```python
from build123d import *

# Parameters (mm, degrees)
SKETCH1_W               = 40
SKETCH1_H               = 35
BOSS_EXTRUDE1_DEPTH     = 8
CUT_EXTRUDE1_DEPTH      = 1
CUT_EXTRUDE1_DEPTH_BACK = 41
FILLET1_R               = 2
SKETCH6_R               = 2
BOSS_EXTRUDE2_DEPTH     = 5
CUT_EXTRUDE2_DEPTH      = 7.467619242
SKETCH6_7_R             = 4.25
CUT_EXTRUDE3_DEPTH      = 3
SKETCH7_W               = 10
SKETCH7_H               = 3
CUT_EXTRUDE4_DEPTH      = 3
FILLET2_R               = 1
SKETCH8_W               = 20
SKETCH8_H               = 2
CUT_EXTRUDE5_DEPTH      = 36
SKETCH10_R              = 4.25
SKETCH10_R_2            = 2
SKETCH10_R_3            = 9
CUT_EXTRUDE6_DEPTH      = 3
FILLET3_R               = 0.5
SKETCH5_W               = 35
SKETCH5_H               = 2
BOSS_EXTRUDE3_DEPTH     = 10
SKETCH12_R              = 2
CUT_EXTRUDE7_DEPTH      = 7.467619242


with BuildPart() as part:
    # Sketch1 → Boss-Extrude1 (new body)
    with BuildSketch(Plane(origin=(0, 0, 0), x_dir=(1, 0, 0), z_dir=(0, 1, 0))):
        Rectangle(SKETCH1_W, SKETCH1_H)
    extrude(amount=-BOSS_EXTRUDE1_DEPTH)

    # Sketch2 → Cut-Extrude1 (cut, two sides)
    with BuildSketch(Plane(origin=(20, 0, 0), x_dir=(0, 0, -1), z_dir=(1, 0, 0))) as cut_extrude1_sk:
        Polygon((-12.5, -5), (-17.5, -8), (0, -8), (0, -5), align=None)
        Polygon((0, -5), (0, -8), (17.5, -8), (12.5, -5), align=None)
    extrude(amount=CUT_EXTRUDE1_DEPTH, mode=Mode.SUBTRACT)
    extrude(cut_extrude1_sk.sketch, amount=-CUT_EXTRUDE1_DEPTH_BACK, mode=Mode.SUBTRACT)

    # Fillet1
    fillet1_edges = [part.edges().sort_by_distance(p)[0] for p in [
        (0, -8, -17.5),
        (0, -5, 12.5),
        (0, -5, -12.5),
        (0, -8, 17.5),
    ]]
    fillet(fillet1_edges, radius=FILLET1_R)

    # Sketch6 → Boss-Extrude2 (add)
    with BuildSketch(Plane(origin=(0, 0, 0), x_dir=(1, 0, 0), z_dir=(0, 1, 0))):
        with BuildLine():
            Line((20, 17.5), (20, -17.5))
            Line((20, -17.5), (40, -17.5))
            ThreePointArc((40, -17.5), (57.5, 0), (40, 17.5))
            Line((40, 17.5), (20, 17.5))
        make_face()
        with Locations((40, -12)):
            Circle(SKETCH6_R, mode=Mode.SUBTRACT)
        with BuildLine():
            ThreePointArc((37.420408929, -8.622395833), (40, -7.75), (42.579591071, -8.622395833))
            ThreePointArc((42.579591071, -8.622395833), (40, -9), (37.420408929, -8.622395833))
        make_face(mode=Mode.SUBTRACT)
        with BuildLine():
            ThreePointArc((31.377604167, -2.579591071), (31, 0), (31.377604167, 2.579591071))
            ThreePointArc((31.377604167, 2.579591071), (32.025997871, 1.361558352), (32.25, 0))
            ThreePointArc((32.25, 0), (32.025997871, -1.361558352), (31.377604167, -2.579591071))
        make_face(mode=Mode.SUBTRACT)
        with BuildLine():
            ThreePointArc((37.420408929, 8.622395833), (40, 9), (42.579591071, 8.622395833))
            ThreePointArc((42.579591071, 8.622395833), (40, 7.75), (37.420408929, 8.622395833))
        make_face(mode=Mode.SUBTRACT)
        with Locations((40, 12)):
            Circle(SKETCH6_R, mode=Mode.SUBTRACT)
        with BuildLine():
            ThreePointArc((48.622395833, -2.579591071), (47.75, 0), (48.622395833, 2.579591071))
            ThreePointArc((48.622395833, 2.579591071), (49, 0), (48.622395833, -2.579591071))
        make_face(mode=Mode.SUBTRACT)
    extrude(amount=-BOSS_EXTRUDE2_DEPTH)

    # Sketch6<6> → Cut-Extrude2 (cut, through all)
    with BuildSketch(Plane(origin=(0, 0, 0), x_dir=(1, 0, 0), z_dir=(0, 1, 0))):
        with BuildLine():
            ThreePointArc((37.420408929, 8.622395833), (33.636038969, 6.363961031), (31.377604167, 2.579591071))
            ThreePointArc((31.377604167, 2.579591071), (32.025997871, 1.361558352), (32.25, 0))
            ThreePointArc((32.25, 0), (32.025997871, -1.361558352), (31.377604167, -2.579591071))
            ThreePointArc((31.377604167, -2.579591071), (33.636038969, -6.363961031), (37.420408929, -8.622395833))
            ThreePointArc((37.420408929, -8.622395833), (40, -7.75), (42.579591071, -8.622395833))
            ThreePointArc((42.579591071, -8.622395833), (46.363961031, -6.363961031), (48.622395833, -2.579591071))
            ThreePointArc((48.622395833, -2.579591071), (47.75, 0), (48.622395833, 2.579591071))
            ThreePointArc((48.622395833, 2.579591071), (46.363961031, 6.363961031), (42.579591071, 8.622395833))
            ThreePointArc((42.579591071, 8.622395833), (40, 7.75), (37.420408929, 8.622395833))
        make_face()
    extrude(amount=-CUT_EXTRUDE2_DEPTH, mode=Mode.SUBTRACT)

    # Sketch6<7> → Cut-Extrude3 (cut)
    with BuildSketch(Plane(origin=(0, 0, 0), x_dir=(1, 0, 0), z_dir=(0, 1, 0))):
        with Locations((52, 0)):
            Circle(SKETCH6_7_R)
        with Locations((28, 0)):
            Circle(SKETCH6_7_R)
    extrude(amount=-CUT_EXTRUDE3_DEPTH, mode=Mode.SUBTRACT)

    # Sketch7 → Cut-Extrude4 (cut)
    with BuildSketch(Plane(origin=(0, 0, 0), x_dir=(1, 0, 0), z_dir=(0, 1, 0))):
        with Locations((29, -16)):
            Rectangle(SKETCH7_W, SKETCH7_H)
    extrude(amount=-CUT_EXTRUDE4_DEPTH, mode=Mode.SUBTRACT)

    # Fillet2
    fillet2_edges = [part.edges().sort_by_distance(p)[0] for p in [
        (34, -1.5, 17.5),
    ]]
    fillet(fillet2_edges, radius=FILLET2_R)

    # Sketch8 → Cut-Extrude5 (cut, through all)
    with BuildSketch(Plane.XY.offset(17.5)):
        with Locations((12, -1)):
            Rectangle(SKETCH8_W, SKETCH8_H)
    extrude(amount=-CUT_EXTRUDE5_DEPTH, mode=Mode.SUBTRACT)

    # Sketch10 → Cut-Extrude6 (cut)
    with BuildSketch(Plane.XZ.offset(5)):
        with Locations((40, -12)):
            Circle(SKETCH10_R)
        with Locations((40, -12)):
            Circle(SKETCH10_R_2, mode=Mode.SUBTRACT)
        with Locations((40, 0)):
            Circle(SKETCH10_R_3)
        with Locations((40, 12)):
            Circle(SKETCH10_R)
        with Locations((40, 12)):
            Circle(SKETCH10_R_2, mode=Mode.SUBTRACT)
        with Locations((40, 0)):
            Circle(SKETCH10_R_3)
    extrude(amount=-CUT_EXTRUDE6_DEPTH, mode=Mode.SUBTRACT)

    # Fillet3
    fillet3_edges = [part.edges().sort_by_distance(p)[0] for p in [
        (49, -5, 0),
        (40, -5, -16.25),
        (40, -5, 16.25),
        (31, -5, 0),
    ]]
    fillet(fillet3_edges, radius=FILLET3_R)

    # Sketch5 → Boss-Extrude3 (add)
    with BuildSketch(Plane.ZY.offset(20)):
        with Locations((0, -1)):
            Rectangle(SKETCH5_W, SKETCH5_H)
    extrude(amount=BOSS_EXTRUDE3_DEPTH)

    # Sketch12 → Cut-Extrude7 (cut, through all)
    with BuildSketch(Plane(origin=(0, 0, 0), x_dir=(1, 0, 0), z_dir=(0, 1, 0))):
        with Locations((-25, 12)):
            Circle(SKETCH12_R)
        with Locations((-25, -12)):
            Circle(SKETCH12_R)
    extrude(amount=-CUT_EXTRUDE7_DEPTH, mode=Mode.SUBTRACT)


solid = part.part
```
Input: part model. Units: mm. Frame: model coordinates. A direction names the side the tool comes from. Coordinates: 2 decimals unless noted, no trailing zeros. Order: outer loops, then holes, each group sorted by start corner. A loop starts at its lowest first (then second) coordinate and runs counter-clockwise, first axis right, second up. Notation, with made-up numbers: (81.5, 70) - (90.5, 70) arc R9 ccw to (90.5, 78) - close; hole circle Ø1 at (-26.5, -0.5). An arc over 180 degrees is marked (long way). Put each result on its own line as item: value.
1. Line query: line 1 along Z through (x, y) = (40, -4); line 2 along Z through (x, y) = (40, -0.95); line 3 along X through (y, z) = (-1.15, -12). Output: solid intervals per line, ascending.
Report:
line 1: z = -17.5 to -16.25, 16.25 to 17.5
line 2: z = -17.5 to -14, -10 to -9, 9 to 10, 14 to 17.5
line 3: x = -30 to -27, -23 to 2, 22 to 38, 42 to 52.74
2. Cut plane C-C on x = 13.5. Return the cut outline in (y, z).
Report:
outline: (-6.18, -14.47) arc R2 ccw to (-4.47, -17.5) - (-2, -17.5) - (-2, 17.5) - (-4.47, 17.5) arc R2 ccw to (-6.18, 14.47) - (-5.29, 12.98) arc R2 cw to (-5, 11.95) - (-5, -11.95) arc R2 cw to (-5.29, -12.98) - close
3. Contact query for flat-ended pins moving along their axis: pin 1 Ø2.5 at (x, y) = (28.5, -1.5) entering from +Z; pin 2 Ø10 at (x, z) = (15.5, 6.5) entering from +Y; pin 3 Ø1.5 at (y, z) = (-3.5, 4) entering from +X. Output: stop coordinate, or through.
Report:
pin 1: stops at z = 14.5
pin 2: stops at y = -2
pin 3: stops at x = 57.2
4. Cut plane A-A on x = -5. Return the cut outline in (y, z), then the cut area to 3 significant figures.
Report:
outline: (-6.18, -14.47) arc R2 ccw to (-4.47, -17.5) - (0, -17.5) - (0, 17.5) - (-4.47, 17.5) arc R2 ccw to (-6.18, 14.47) - (-5.29, 12.98) arc R2 cw to (-5, 11.95) - (-5, -11.95) arc R2 cw to (-5.29, -12.98) - close
area: 184 mm2
5. Draft query along Z for faces 1 (the face through (22, -1, 0)), 2 (the face through (0.28, -5.74, -13.73)), 3 (the face through (18, -5, 0)), 4 (the face through (57.496, -2.465, 0.385)). Return one class per face: pulls with the +Z half, pulls with the -Z half, needs draft (parallel to the pull), parting line crosses it, or undercut.
Report:
face 1: needs draft
face 2: undercut
face 3: undercut
face 4: parting line crosses it
6. Cut plane B-B on x = 50.5. Return the cut outline in (y, z), then the cut area to 3 significant figures.
Report:
outline: (-5, -14) - (0, -14) - (0, -3.98) - (-3, -3.98) - (-3, 3.98) - (0, 3.98) - (0, 14) - (-5, 14) - close
area: 116 mm2
7. Reachability of faces 5 (the face through (0.28, -5.728, 13.713)), 6 (the face through (12, -2, 0)), 7 (the face through (-25, -2, 0)) from +Z, -Z, +X, -X, +Y, -Y: full face, straight path, thin tool, end or side. Return the list, or none.
Report:
face 5: +X, -X, -Y
face 6: +Z, -Z, +Y
face 7: +Z, -Z, -X, -Y
